Here's how the part is built. I have some questions about the finished solid (model axes, mm). A direction names the side the tool comes from. Round coordinates to 2 decimals unless told otherwise and drop trailing zeros. Write each loop counter-clockwise with the first axis right and the second up, starting at its lowest first coordinate (ties: lowest second). Pieces come first, ordered by that corner, then holes. Notation, with made-up numbers: (10, -24) -> (23, -24) arc R17 cw to (23, 9) -> close; hole circle Ø10 at (-25.75, 8.25). An arc over 180 degrees is marked (long way). Put each result on its own line as item: value. Start each with the question number.
1) Which directions (+Z, -Z, +X, -X, +Y, -Y) give clear straight access to the entire face, cutting with the end or side of a thin tool? Please do faces 4 (the flat face through (0, 4.089, 4)), 5 (the flat face through (-4.3, 0.1, 1.778)), 6 (the flat face through (6, 0, 6.35)).
2) If I drill on line 1 along Z through (x, y) = (-7, -3.5); line 2 along Y through (x, z) = (0, 1.05); line 3 along X through (y, z) = (-1, 5.75), over which ranges is the centre line in solid material (lowest first)? Write a range as [from, to].
3) I want a section at A-A, the plane z = 2.5. List the corners of the cut face in (x, y) for me, then the cut area to 3 significant figures.
4) We'd pull the mould along Y, two halves only. Please class faces 1 (the flat face through (-21.7, 13.2, 3.1)), 2 (the flat face through (-4.089, 0, 4)), 3 (the flat face through (13, 0, 0)): released by +Y, released by -Y, zero draft, split by the parting line, or undercut.
5) Will these pins go through, and if not, where does the flat tip stop? P1, Ø2.5, axis at x = 2, z = 3.5, coming from the -Y side; P2, Ø3.5, axis at x = 1.5, z = 5, coming from the +Y side; P3, Ø1.5, axis at x = 22, z = 5, coming from the -Y side.
6) I want a section at C-C, the plane x = 5. List the corners of the cut face in (y, z) for me, then the cut area to 3 significant figures.
7) I want a section at B-B, the plane y = -5. List the corners of the cut face in (x, z) for me.
8) I want a section at D-D, the plane y = 20. List the corners of the cut face in (x, z) for me, then the cut area to 3 significant figures.
from build123d import *

# Parameters (mm, degrees)
F0_R     = 9.271
F0_W     = 8.1788
F0_H     = 8.1788
F1_DEPTH = 6.35
F2_DEPTH = 1.778


with BuildPart() as f1:
    # F0 (on Top) → F1 (new body)
    with BuildSketch(Plane.XY):
        with BuildLine():
            ThreePointArc((21.7969618714, -13.0404161427), (24.4826758294, -6.7645091642), (25.4, 0))
            ThreePointArc((25.4, 0), (24.5848737642, 6.3831012839), (22.1918124409, 12.3565149045))
            ThreePointArc((22.1918124409, 12.3565149045), (13.0404159786, 21.7969619696), (0.3948506462, 25.3969307785))
            ThreePointArc((0.3948506462, 25.3969307785), (-12.3565148847, 22.191812452), (-21.7969621275, 13.0404157147))
            ThreePointArc((-21.7969621275, 13.0404157147), (-25.3969307892, 0.3948499567), (-22.1918120914, -12.3565155323))
            ThreePointArc((-22.1918120914, -12.3565155323), (-13.0404155443, -21.7969622294), (-0.3948503527, -25.396930783))
            ThreePointArc((-0.3948503527, -25.396930783), (12.356514795, -22.1918125019), (21.7969618714, -13.0404161427))
        make_face()
        Circle(F0_R, mode=Mode.SUBTRACT)
        with BuildLine():
            ThreePointArc((-21.7969621275, 13.0404157147), (-12.3565148847, 22.191812452), (0.3948506462, 25.3969307785))
            Line((0.3948506462, 25.3969307785), (-14.2680745061, 25.6248977212))
            Line((-14.2680745061, 25.6248977212), (-21.7969621275, 13.0404157147))
        make_face()
        with BuildLine():
            ThreePointArc((0.3948506462, 25.3969307785), (13.0404159786, 21.7969619696), (22.1918124409, 12.3565149045))
            Line((22.1918124409, 12.3565149045), (15.0577751429, 25.168963846))
            Line((15.0577751429, 25.168963846), (0.3948506462, 25.3969307785))
        make_face()
        with BuildLine():
            ThreePointArc((22.1918124409, 12.3565149045), (24.5848737642, 6.3831012839), (25.4, 0))
            ThreePointArc((25.4, 0), (24.4826758294, -6.7645091642), (21.7969618714, -13.0404161427))
            Line((21.7969618714, -13.0404161427), (29.325849649, -0.4559338752))
            Line((29.325849649, -0.4559338752), (22.1918124409, 12.3565149045))
        make_face()
        with BuildLine():
            Line((14.2680745061, -25.6248977212), (21.7969618714, -13.0404161427))
            ThreePointArc((21.7969618714, -13.0404161427), (12.356514795, -22.1918125019), (-0.3948503527, -25.396930783))
            Line((-0.3948503527, -25.396930783), (14.2680745061, -25.6248977212))
        make_face()
        with BuildLine():
            Line((-15.0577751429, -25.168963846), (-0.3948503527, -25.396930783))
            ThreePointArc((-0.3948503527, -25.396930783), (-13.0404155443, -21.7969622294), (-22.1918120914, -12.3565155323))
            Line((-22.1918120914, -12.3565155323), (-15.0577751429, -25.168963846))
        make_face()
        with BuildLine():
            ThreePointArc((-22.1918120914, -12.3565155323), (-25.3969307892, 0.3948499567), (-21.7969621275, 13.0404157147))
            Line((-21.7969621275, 13.0404157147), (-29.325849649, 0.4559338752))
            Line((-29.325849649, 0.4559338752), (-22.1918120914, -12.3565155323))
        make_face()
        Circle(F0_R)
        Rectangle(F0_W, F0_H, mode=Mode.SUBTRACT)
    extrude(amount=F1_DEPTH)

    # F0 (on Top) → F2 (cut)
    with BuildSketch(Plane.XY):
        Circle(F0_R)
        Rectangle(F0_W, F0_H, mode=Mode.SUBTRACT)
    extrude(amount=F2_DEPTH, mode=Mode.SUBTRACT)


solid = f1.part
Findings:
1. face 4: +Z, -Z
1. face 5: -Z
1. face 6: +Z, +X, -X, +Y, -Y
2. line 1: z = [1.78, 6.35]
2. line 2: y = [-25.4, -9.27], [9.27, 25.4]
2. line 3: x = [-28.52, -4.09], [4.09, 29]
3. outline: (-29.33, 0.46) -> (-15.06, -25.17) -> (14.27, -25.62) -> (29.33, -0.46) -> (15.06, 25.17) -> (-14.27, 25.62) -> close; hole (-4.09, -4.09) -> (4.09, -4.09) -> (4.09, 4.09) -> (-4.09, 4.09) -> close
3. area: 2,170 mm2
4. face 1: released by +Y
4. face 2: undercut
4. face 3: zero draft
5. P1: stops at y = -25.45
5. P2: stops at y = 25.41
5. P3: stops at y = -13.95
6. outline: (-25.48, 0) -> (-7.81, 0) -> (-7.81, 1.78) -> (7.81, 1.78) -> (7.81, 0) -> (25.33, 0) -> (25.33, 6.35) -> (-25.48, 6.35) -> close
6. area: 295 mm2
7. outline: (-26.29, 0) -> (-7.81, 0) -> (-7.81, 1.78) -> (7.81, 1.78) -> (7.81, 0) -> (26.61, 0) -> (26.61, 6.35) -> (-26.29, 6.35) -> close
8. outline: (-17.63, 0) -> (17.94, 0) -> (17.94, 6.35) -> (-17.63, 6.35) -> close
8. area: 226 mm2
